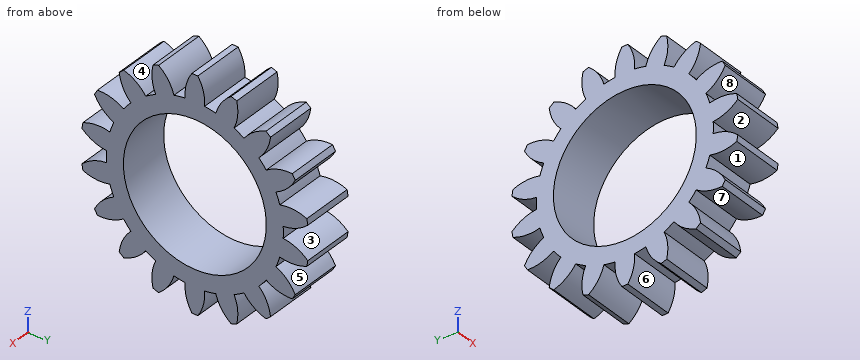
from build123d import *

# Parameters (mm, degrees)
BASPROSKE_W             = 8
BASPROSKE_H             = 17.5
TOOTHCUT_DEPTH          = 27.009613607
TEETHCUTS_COUNT         = 18
TEETHCUTS_ANGLE         = 340
BORSKE_R                = 4
BORE_DEPTH              = 50.0000508
ESQUISSE1_R             = 10.95
ENL_V_MAT_EXTRU_1_DEPTH = 10


with BuildPart() as part:
    # BasProSke → Base-Revolve (revolve)
    with BuildSketch(Plane(origin=(0, 0, 0), x_dir=(1, 0, 0), z_dir=(0, 1, 0)), mode=Mode.PRIVATE) as base_revolve_sk:
        with Locations((4, 8.75)):
            Rectangle(BASPROSKE_W, BASPROSKE_H)
    revolve(base_revolve_sk.sketch.rotate(Axis((-10, 0, 0), (1, 0, 0)), 180), axis=Axis((-10, 0, 0), (1, 0, 0)))

    # TooCutSke → ToothCut (cut, through all)
    with BuildSketch(Plane(origin=(0, 0, 0), x_dir=(0, 0, -1), z_dir=(1, 0, 0))):
        with BuildLine():
            ThreePointArc((0.873326889, 13.533350745), (0, 13.5615), (-0.873326889, 13.533350745))
            ThreePointArc((-0.873326889, 13.533350745), (-1.417662776, 15.579682129), (-2.609262071, 17.330072031))
            ThreePointArc((-2.609262071, 17.330072031), (0, 17.5254), (2.609262071, 17.330072031))
            ThreePointArc((2.609262071, 17.330072031), (1.417662776, 15.579682129), (0.873326889, 13.533350745))
        make_face()
    toothcut = extrude(amount=TOOTHCUT_DEPTH, mode=Mode.SUBTRACT)

    # TeethCuts: ToothCut ×18 about axis
    teethcuts_axis = Axis((-10, 0, 0), (1, 0, 0))
    for i in range(1, TEETHCUTS_COUNT):
        add(toothcut.rotate(teethcuts_axis, i * TEETHCUTS_ANGLE / (TEETHCUTS_COUNT - 1)), mode=Mode.SUBTRACT)

    # BorSke → Bore (cut, symmetric)
    with BuildSketch(Plane(origin=(0, 0, 0), x_dir=(0, 0, -1), z_dir=(1, 0, 0))):
        with Locations(Location((0, 0, 0), (0, 0, 180))):
            Circle(BORSKE_R)
    extrude(amount=BORE_DEPTH, both=True, mode=Mode.SUBTRACT)

    # Esquisse1 → Enlèv. mat.-Extru.1 (cut)
    with BuildSketch(Plane(origin=(8, 0, 0), x_dir=(0, 0, -1), z_dir=(1, 0, 0))):
        Circle(ESQUISSE1_R)
    extrude(amount=-ENL_V_MAT_EXTRU_1_DEPTH, mode=Mode.SUBTRACT)


solid = part.part
CAD build for the part. Positions are in the model's coordinates, mm. Face numbers are marked on the shaded views. A direction names the side the tool comes from. Give positions to 0.01 mm unless a question says otherwise; leave off trailing zeros. Loops run counter-clockwise (first coordinate to the right, second up) from the corner with the lowest first, then second, coordinate; pieces in that order, holes last. Notation, with made-up numbers: M 52.25,-23.5 L 76.25,-23.5 A20 ccw 76.25,-17.5 Z; hole C 64,42 d5. An arc over 180 degrees is marked long. Write each question's results on one line, items separated by ' | '.
Q1. Band-saw the part on A-A on y = 0. Write the cut outline in (x, z).
Geometry check:
outline: M 0,-17.5 L 8,-17.5 L 8,-10.95 L 0,-10.95 Z; M 0,10.95 L 8,10.95 L 8,17.5 L 0,17.5 Z
Q2. Mould opens along Y. For the marked faces 5, 6, 7 and 8 say: pulls with the +Y half, pulls with the -Y half, needs draft (parallel to the pull), parting line crosses it, or undercut.
Geometry check:
face 5: pulls with the +Y half | face 6: undercut | face 7: undercut | face 8: pulls with the -Y half
Q3. Flat gauge pins, fed straight in: P1, Ø2, axis at x = 6.5, y = 12.5, coming from the +Z side; P2, Ø3, axis at x = 4.5, y = -12.5, coming from the -Z side; P3, Ø1, axis at x = 5, y = -1, coming from the +Z side. Where does each tip first touch, or does it go through?
Geometry check:
P1: stops at z = 13.19 | P2: stops at z = -13.61 | P3: stops at z = 17.43
Q4. Probe probe 1 along Y at (x, z) = (6.25, 0); probe 2 along Z at (x, y) = (7, 14.5); probe 3 along Y at (x, z) = (4, 2.5). List the from-to ranges inside material, lowest first.
Geometry check:
probe 1: y = -13.56 to -10.95, 10.95 to 13.56 | probe 2: z = -9.16 to -7.03, -4.02 to -1.04, 1.04 to 4.02, 7.03 to 9.16 | probe 3: y = -17.21 to -10.66, 10.66 to 17.21
Q5. Which spindle directions (+Z, -Z, +X, -X, +Y, -Y) get a long thin tool onto all of the face, cutting with end or side? Do the marked faces 1, 2, 3 and 4. Say none if no direction does.
Geometry check:
face 1: +X, -X | face 2: +X, -X, -Y | face 3: +X, -X, +Y | face 4: +Z, +X, -X
Q6. Band-saw the part on B-B on z = 0. Write the cut outline in (x, y), and give its area (3 significant figures).
Geometry check:
outline: M 0,-13.56 L 8,-13.56 L 8,-10.95 L 0,-10.95 Z; M 0,10.95 L 8,10.95 L 8,13.56 L 0,13.56 Z | area: 41.8 mm²
